Read the model definition and answer for the solid it produces. Units are mm, in the model's axes. Face numbers are marked on the shaded views. A direction names the side the tool comes from. Round coordinates to 2 decimals unless told otherwise and drop trailing zeros. Loops run counter-clockwise (first coordinate to the right, second up) from the corner with the lowest first, then second, coordinate; pieces in that order, holes last. Notation, with made-up numbers: M 78.25,-0.75 L 89.25,-0.75 A25 ccw 89.25,20.25 Z; hole C 28.25,22 d1. An arc over 180 degrees is marked long. Write each question's results on one line, items separated by ' | '.
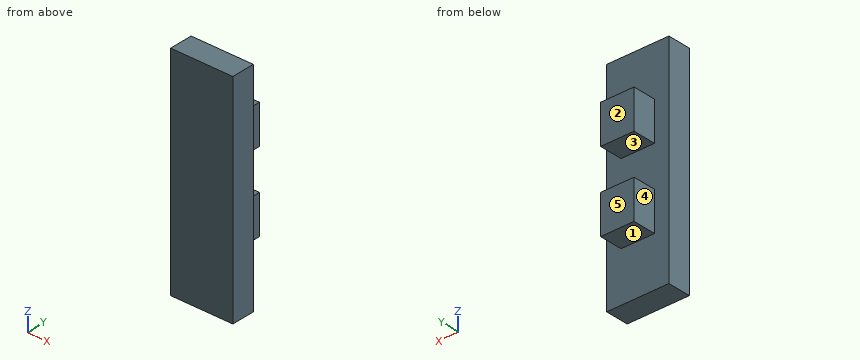
```python
from build123d import *

# Parameters (mm, degrees)
F0_W     = 80
F0_H     = 280
F1_DEPTH = 30
F3_START = 26
F2_W     = 43
F2_H     = 30
F3_DEPTH = 50
F4_START = -26
F4_DEPTH = 50


with BuildPart() as f1:
    # F0 (on Front) → F1 (new body)
    with BuildSketch(Plane.XZ):
        Rectangle(F0_W, F0_H)
    extrude(amount=F1_DEPTH)

    # F2 (on Top) → F3 (join)
    with BuildSketch(Plane.XY.offset(F3_START)):
        with Locations((0, 15)):
            Rectangle(F2_W, F2_H)
    extrude(amount=F3_DEPTH)

    # F2 (on Top) → F4 (join)
    with BuildSketch(Plane.XY.offset(F4_START)):
        with Locations((0, 15)):
            Rectangle(F2_W, F2_H)
    extrude(amount=-F4_DEPTH)


solid = f1.part
```
1. Find section B-B, the plane z = -35.5. Give the vertices of the cut face in (x, y).
Completed:
outline: M -40,-30 L 40,-30 L 40,0 L 21.5,0 L 21.5,30 L -21.5,30 L -21.5,0 L -40,0 Z
2. Given P1, Ø15, axis at x = -2, y = 11, coming from the -Z side; P2, Ø24, axis at y = 21, z = -56.5, coming from the +X side; P3, Ø8, axis at x = -14.5, z = -101.5, coming from the +Y side, each flat-ended and moving along its own axis, determine where each tip first touches the part or whether it passes through.
Completed:
P1: stops at z = -76 | P2: stops at x = 21.5 | P3: stops at y = 0
3. Find the intervals of material crossed by L1, parallel to Z at x = 7.5, y = 23.5; L2, parallel to Y at x = -36, z = 73; L3, parallel to X at y = 2.5, z = 57, in increasing order.
Completed:
L1: z = -76 to -26, 26 to 76 | L2: y = -30 to 0 | L3: x = -21.5 to 21.5
4. Find section D-D, the plane x = -35. Give the vertices of the cut face in (y, z).
Completed:
outline: M -30,-140 L 0,-140 L 0,140 L -30,140 Z
5. Find section A-A, the plane y = 9. Give the vertices of the cut face in (x, z).
Completed:
outline: M -21.5,-76 L 21.5,-76 L 21.5,-26 L -21.5,-26 Z; M -21.5,26 L 21.5,26 L 21.5,76 L -21.5,76 Z
6. Which of the six approach directions +Z, -Z, +X, -X, +Y, -Y give full straight-line access (tool end or side, diameter ignored) to the marked faces 4 and 5?
Completed:
face 4: +Z, -Z, -X, +Y | face 5: +Z, -Z, +X, -X, +Y
7. Find section C-C, the plane x = 15. Give the vertices of the cut face in (y, z), then the cut area to 3 significant figures.
Completed:
outline: M -30,-140 L 0,-140 L 0,-76 L 30,-76 L 30,-26 L 0,-26 L 0,26 L 30,26 L 30,76 L 0,76 L 0,140 L -30,140 Z | area: 11,400 mm2
8. Determine the mould class of the marked faces 1, 2 and 3 for opening direction Z: released by +Z, released by -Z, zero draft, split by the parting line, or undercut.
Completed:
face 1: released by -Z | face 2: zero draft | face 3: undercut
